from build123d import *

# Parameters (mm, degrees)
F1_DEPTH = 4.763
F2_D     = 2.5
F3_D     = 4
F4_D     = 6
F5_D     = 12


with BuildPart() as f1:
    # F0 (on Right) → F1 (new body)
    with BuildSketch(Plane.YZ):
        Polygon((30, 17), (22, 17), (-17.5, 17), (-27.5, 17), (-27.5, 0), (-27.5, -17), (-17.5, -17), (22, -17), (30, -17), (30, 0), align=None)
        with BuildLine():
            Line((22, 35), (22, 17))
            Line((22, 17), (30, 17))
            Line((30, 17), (30, 18))
            ThreePointArc((30, 18), (31.4644660941, 21.5355339059), (35, 23))
            Line((35, 23), (41, 23))
            ThreePointArc((41, 23), (44.5355339059, 21.5355339059), (46, 18))
            Line((46, 18), (46, 17))
            Line((46, 17), (58.5, 17))
            Line((58.5, 17), (58.5, 45))
            Line((58.5, 45), (32, 45))
            Line((32, 45), (22, 35))
        make_face()
        with BuildLine():
            Line((-27.5, 17), (-17.5, 17))
            Line((-17.5, 17), (-17.5, 38))
            Line((-17.5, 38), (-15.5, 38))
            Line((-15.5, 38), (-15.5, 50))
            Line((-15.5, 50), (-21, 50))
            Line((-21, 50), (-53, 50))
            Line((-53, 50), (-58.5, 50))
            Line((-58.5, 50), (-58.5, 38))
            Line((-58.5, 38), (-58.5, 17))
            Line((-58.5, 17), (-48.5, 17))
            Line((-48.5, 17), (-48.5, 35))
            ThreePointArc((-48.5, 35), (-47.0355339059, 38.5355339059), (-43.5, 40))
            Line((-43.5, 40), (-32.5, 40))
            ThreePointArc((-32.5, 40), (-28.9644660941, 38.5355339059), (-27.5, 35))
            Line((-27.5, 35), (-27.5, 17))
        make_face()
        Polygon((58.5, 17), (46, 17), (46, 0), (46, -17), (58.5, -17), align=None)
        Polygon((-48.5, 0), (-48.5, 17), (-58.5, 17), (-58.5, -17), (-48.5, -17), align=None)
        with BuildLine():
            Line((30, -18), (30, -17))
            Line((30, -17), (22, -17))
            Line((22, -17), (22, -35))
            Line((22, -35), (32, -45))
            Line((32, -45), (58.5, -45))
            Line((58.5, -45), (58.5, -17))
            Line((58.5, -17), (46, -17))
            Line((46, -17), (46, -18))
            ThreePointArc((46, -18), (44.5355339059, -21.5355339059), (41, -23))
            Line((41, -23), (35, -23))
            ThreePointArc((35, -23), (31.4644660941, -21.5355339059), (30, -18))
        make_face()
        with BuildLine():
            Line((-17.5, -17), (-27.5, -17))
            Line((-27.5, -17), (-27.5, -35))
            ThreePointArc((-27.5, -35), (-28.9644660941, -38.5355339059), (-32.5, -40))
            Line((-32.5, -40), (-43.5, -40))
            ThreePointArc((-43.5, -40), (-47.0355339059, -38.5355339059), (-48.5, -35))
            Line((-48.5, -35), (-48.5, -17))
            Line((-48.5, -17), (-58.5, -17))
            Line((-58.5, -17), (-58.5, -38))
            Line((-58.5, -38), (-58.5, -50))
            Line((-58.5, -50), (-53, -50))
            Line((-53, -50), (-21, -50))
            Line((-21, -50), (-15.5, -50))
            Line((-15.5, -50), (-15.5, -38))
            Line((-15.5, -38), (-17.5, -38))
            Line((-17.5, -38), (-17.5, -17))
        make_face()
    extrude(amount=F1_DEPTH)

    # F2 (through all)
    with Locations(Plane(origin=(0, 0, 0), x_dir=(0, 1, 0), z_dir=(-1, 0, 0))):
        with Locations((-53, -45), (-21, -45), (-21, 45), (-53, 45)):
            Hole(F2_D / 2)

    # F3 (through all)
    with Locations(Plane(origin=(0, 0, 0), x_dir=(0, 1, 0), z_dir=(-1, 0, 0))):
        with Locations((-9, -10), (15, -10), (15, 10), (-9, 10)):
            Hole(F3_D / 2)

    # F4 (through all)
    with Locations(Plane(origin=(0, 0, 0), x_dir=(0, 1, 0), z_dir=(-1, 0, 0))):
        with Locations((52, 0), (28.5, 29.5), (28.5, -29.5)):
            Hole(F4_D / 2)

    # F5 (through all)
    with Locations(Plane(origin=(0, 0, 0), x_dir=(0, 1, 0), z_dir=(-1, 0, 0))):
        with Locations((41, -35), (41, 35)):
            Hole(F5_D / 2)


solid = f1.part
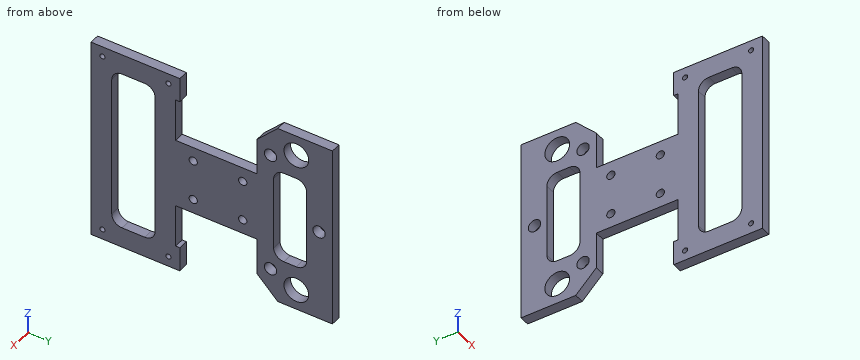
Geometry: final body of the model. Coordinates: model frame, mm. Round coordinates to 2 decimals unless told otherwise and drop trailing zeros. Loops run counter-clockwise (first coordinate to the right, second up) from the corner with the lowest first, then second, coordinate; pieces in that order, holes last.
Q1. Material intervals for L1, parallel to Z at x = 2.7, y = -53; L2, parallel to Y at x = 4.1, z = -16; L3, parallel to Z at x = 3.7, y = 15, sorted ascending.
Q2. Section A-A on y = -9. Return loops of the section in (x, z), plus the area to 3 significant figures.
Q3. Section B-B on z = -6. Return loops of the section in (x, y), plus the area to 3 significant figures.
Q4. Section C-C on y = -47. Return loops of the section in (x, z), plus the area to 3 significant figures.
Q5. Pin query (flat end, axial travel): P1, Ø3, axis at y = -9, z = -10, coming from the +X side; P2, Ø3, axis at y = -53, z = 45, coming from the +X side. Return the tip coordinate at first contact, or that it passes through.
Q6. Section D-D on x = 1.15. State how many separate pieces and enclosed holes the cut face has, plus the area to 3 significant figures.
Evaluation:
1. L1: z = -50 to -46.25, -43.75 to 43.75, 46.25 to 50
1. L2: y = -58.5 to -48.5, -27.5 to 30, 46 to 58.5
1. L3: z = -17 to -12, -8 to 8, 12 to 17
2. outline: (0, -17) - (4.76, -17) - (4.76, -12) - (0, -12) - close; (0, -8) - (4.76, -8) - (4.76, 8) - (0, 8) - close; (0, 12) - (4.76, 12) - (4.76, 17) - (0, 17) - close
2. area: 124 mm2
3. outline: (0, -58.5) - (4.76, -58.5) - (4.76, -48.5) - (0, -48.5) - close; (0, -27.5) - (4.76, -27.5) - (4.76, 30) - (0, 30) - close; (0, 46) - (4.76, 46) - (4.76, 58.5) - (0, 58.5) - close
3. area: 381 mm2
4. outline: (0, -50) - (4.76, -50) - (4.76, -38.57) - (0, -38.57) - close; (0, 38.57) - (4.76, 38.57) - (4.76, 50) - (0, 50) - close
4. area: 109 mm2
5. P1: passes through
5. P2: stops at x = 4.76
6. separate pieces: 1
6. enclosed holes: 15
6. area: 5,920 mm2
